Source: CAD feature listing. Evaluate the final solid. Frame: model axes, mm. Face numbers are marked on the shaded views. Coordinates: 2 decimals unless noted, no trailing zeros. Write each loop counter-clockwise with the first axis right and the second up, starting at its lowest first coordinate (ties: lowest second). Pieces come first, ordered by that corner, then holes. Notation, with made-up numbers: (-5, 59.25) -> (49, 59.25) arc R27 cw to (49, 79.25) -> close; hole circle Ø3 at (65.5, 79.25). An arc over 180 degrees is marked (long way). One line per item, written item: value. Start each with the question number.
1. Section query B-B, the plane y = 7.5. Output: boundary loops of the cut face in (x, z).
2. Line query: line 1 (Z direction, x = 25, y = 12); line 2 (X direction, y = 19.5, z = 60); line 3 (X direction, y = 13, z = 60). Output: solid intervals per line, ascending.
3. First-contact query: P1, Ø1.5, axis at x = 7.5, z = 10, coming from the -Y side. Flat tip, straight axial feed; report the tip coordinate or a pass-through.
4. Mould query, pull axis Z, two halves, no side actions, for the marked faces 1, 2, 3 and 4. Classes: released by +Z, released by -Z, zero draft, split by the parting line, or undercut.
5. Section query D-D, the plane y = 25.25. Output: boundary loops of the cut face in (x, z).
6. Section query C-C, the plane z = 60. Output: boundary loops of the cut face in (x, y).
7. Section query A-A, the plane x = -25. Output: boundary loops of the cut face in (y, z).
Autodesk Inventor part; units mm, degrees
ref_plane "YZ Plane" through (0, 0, 0) normal (1, 0, 0) x (0, 1, 0)
ref_plane "XZ Plane" through (0, 0, 0) normal (0, 1, 0) x (-1, 0, 0)
ref_plane "XY Plane" through (0, 0, 0) normal (0, 0, 1) x (1, 0, 0)
sketch "Sketch1" plane through (0, 0, 0) normal (0, 0, 1) x (1, 0, 0)
  arc A0 (15.1987, 5) -> (-15.1987, 5) centre (0, 0) ccw
  line L0 (-15.1987, 5) -> (-35, 5)
  line L1 (-35, 5) -> (-35, 30)
  line L2 (-35, 30) -> (35, 30)
  line L3 (35, 30) -> (35, 5)
  line L4 (35, 5) -> (15.1987, 5)
  line L5 (0, 0) -> (0, 30)
  dimension "d0" = 32
  dimension "d1" = 70
  dimension "d2" = 5
  dimension "d3" = 19.8013
  dimension "d4" = 25
extrude "Extrusion1" add sketch "Sketch1" along normal mid plane 150
sketch "Sketch2" plane through (-35, 30, 75) normal (0, 1, 0) x (1, 0, 0)
  line L0 (0, 150) -> (70, 150) construction
  line L1 (0, 150) -> (0, 0) construction
  line L2 (35, 75) -> (70, 75)
  line L3 (35, 75) -> (35, 150)
  point P0 (10, 135)
  point P1 (60, 135)
  point P2 (10, 15)
  point P3 (60, 15)
  dimension "d7" = 15
  dimension "d8" = 10
hole "Hole1" at (-25, 30, -60) at (25, 30, -60) at (-25, 30, 60) at (25, 30, 60) direction (0, -1, 0) diameter 14 end through all
properties part number "Suspension_Clamp_Cunha"
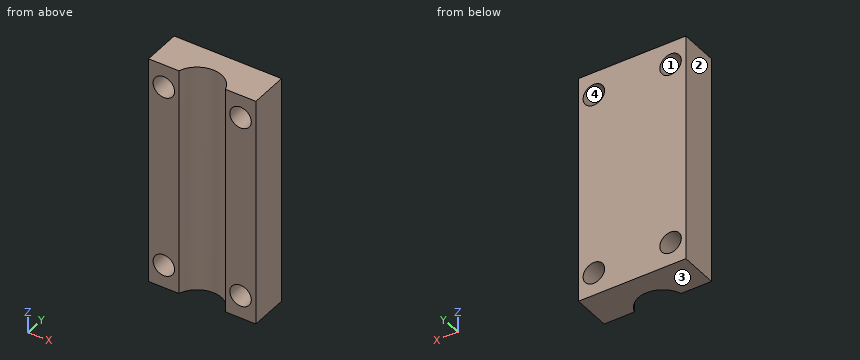
Computed values:
1. outline: (-35, -75) -> (-14.13, -75) -> (-14.13, 75) -> (-35, 75) -> close; (14.13, -75) -> (35, -75) -> (35, 75) -> (14.13, 75) -> close; hole circle Ø14 at (-25, -60); hole circle Ø14 at (-25, 60); hole circle Ø14 at (25, -60); hole circle Ø14 at (25, 60)
2. line 1: z = -75 to -67, -53 to 53, 67 to 75
2. line 2: x = -35 to -32, -18 to 18, 32 to 35
2. line 3: x = -35 to -32, -18 to -9.33, 9.33 to 18, 32 to 35
3. P1: stops at y = 13.71
4. face 1: undercut
4. face 2: zero draft
4. face 3: released by -Z
4. face 4: undercut
5. outline: (-35, -75) -> (35, -75) -> (35, 75) -> (-35, 75) -> close; hole circle Ø14 at (-25, -60); hole circle Ø14 at (-25, 60); hole circle Ø14 at (25, -60); hole circle Ø14 at (25, 60)
6. outline: (-35, 5) -> (-32, 5) -> (-32, 30) -> (-35, 30) -> close; (-18, 5) -> (-15.2, 5) arc R16 cw to (15.2, 5) -> (18, 5) -> (18, 30) -> (-18, 30) -> close; (32, 5) -> (35, 5) -> (35, 30) -> (32, 30) -> close
7. outline: (5, -75) -> (30, -75) -> (30, -67) -> (5, -67) -> close; (5, -53) -> (30, -53) -> (30, 53) -> (5, 53) -> close; (5, 67) -> (30, 67) -> (30, 75) -> (5, 75) -> close
